Geometry check sheet. Reference: the model listing, model coordinates, mm. A direction names the side the tool comes from. Give positions to 0.01 mm unless a question says otherwise; leave off trailing zeros. Write each loop counter-clockwise with the first axis right and the second up, starting at its lowest first coordinate (ties: lowest second). Pieces come first, ordered by that corner, then holes. Notation, with made-up numbers: (81, 37) - (100, 37) arc R15 cw to (100, 56) - close; hole circle Ø5 at (-31.5, -23). An arc over 180 degrees is marked (long way). Write item = value, one per line. Start each with the question number.
(1) Section check D-D, the plane z = -8.75. Enter the section's corners in (x, y), plus the area to 3 significant figures.
(2) Thickness scan on L1, parallel to Y at x = 3.5, z = -1; L2, parallel to Z at x = 2.5, y = -6.25; L3, parallel to Z at x = -2, y = -6. Record the ranges inside material, lowest first.
(3) Section check C-C, the plane y = -7. Enter the section's corners in (x, z) (3 decimals).
(4) Access from +Z, -Z, +X, -X, +Y, -Y to the whole of each face (thin tool, end or side, straight path). Record for faces 1 (the flat face through (-2, -4.762, 3)), 2 (the flat face through (0, 4.762, 0)).
(5) Depth check by flat-ended pin: pin 1 Ø1.5 at (y, z) = (-8.5, -1) entering from -X. Enter the tip coordinate at first touch or a pass-through.
(6) Section check B-B, the plane z = 1. Enter the section's corners in (x, y), plus the area to 3 significant figures.
(7) Section check A-A, the plane x = 0. Enter the section's corners in (y, z) (1 decimal), plus the area to 3 significant figures.
```python
from build123d import *

# Parameters (mm, degrees)
F0_W     = 12.7
F0_H     = 25.4
F1_DEPTH = 4.7625
F2_R     = 3.175
F3_DEPTH = 6.35


with BuildPart() as f1:
    # F0 (on Front) → F1 (new body, symmetric)
    with BuildSketch(Plane.XZ):
        Rectangle(F0_W, F0_H)
    extrude(amount=F1_DEPTH, both=True)

    # F2 (on face) → F3 (join)
    with BuildSketch(Plane.XZ.offset(4.7625)):
        Circle(F2_R)
    extrude(amount=F3_DEPTH)


solid = f1.part
```
Model answer:
q1.outline = (-6.35, -4.76) - (6.35, -4.76) - (6.35, 4.76) - (-6.35, 4.76) - close
q1.area = 121 mm²
q2.L1 = -4.76 to 4.76
q2.L2 = -1.96 to 1.96
q2.L3 = -2.47 to 2.47
q3.outline = circle Ø6.35 at (0, 0)
q4.face_1 = -Y
q4.face_2 = +Z, -Z, +X, -X, +Y
q5.pin_1 = -3.17
q6.outline = (-6.35, -4.76) - (-3.01, -4.76) - (-3.01, -11.11) - (3.01, -11.11) - (3.01, -4.76) - (6.35, -4.76) - (6.35, 4.76) - (-6.35, 4.76) - close
q6.area = 159 mm²
q7.outline = (-11.1, -3.2) - (-4.8, -3.2) - (-4.8, -12.7) - (4.8, -12.7) - (4.8, 12.7) - (-4.8, 12.7) - (-4.8, 3.2) - (-11.1, 3.2) - close
q7.area = 282 mm²
